Here's how the part is built. I have some questions about the finished solid (model axes, mm). A direction names the side the tool comes from. Coordinates: 2 decimals unless noted, no trailing zeros. Write each loop counter-clockwise with the first axis right and the second up, starting at its lowest first coordinate (ties: lowest second). Pieces come first, ordered by that corner, then holes.
(1) Imagine slicing it at A-A, the plane y = -10.5. List the corners of the cut face in (x, z) for me, plus the area to 3 significant figures.
(2) Thinking about a two-plate mould opening in Z: for faces 1 (the flat face through (-2, -15, 5)), 2 (the flat face through (-2, -7, 373)), 3 (the flat face through (117, -5, 114)), which applies, released by +Z, released by -Z, zero draft, split by the parting line, or undercut?
(3) Which directions (+Z, -Z, +X, -X, +Y, -Y) give clear straight access to the entire face, cutting with the end or side of a thin tool? Please do faces 4 (the flat face through (-2, 0, 5)), 5 (the cylindrical face through (117.7, -10.1, 48)).
(4) Please list where these lines run through material, in increasing order: probe 1 along Z at (x, y) = (126, -11.25); probe 2 along X at (y, z) = (-10.5, 58).
(5) For pin 1 Ø8 at (x, z) = (-51.5, 65.5) entering from +Y, with a flat end and sliding along its axis, tell me the tip position at first contact or that it passes through.
(6) Imagine slicing it at B-B, the plane x = 117.5. List the corners of the cut face in (y, z) for me, plus the area to 3 significant figures.
```python
from build123d import *

# Parameters (mm, degrees)
F0_W     = 295
F0_H     = 746
F1_DEPTH = 15
F3_DEPTH = 10


with BuildPart() as f1:
    # F0 (on Front) → F1 (new body)
    with BuildSketch(Plane.XZ):
        Rectangle(F0_W, F0_H)
    extrude(amount=F1_DEPTH)

    # F2 (on face) → F3 (cut)
    with BuildSketch(Plane.XZ.offset(15)):
        with BuildLine():
            ThreePointArc((132.4401133717, 161.6609658553), (132.4850208638, 162.3298136735), (132.5, 163))
            ThreePointArc((132.5, 163), (116.3496874374, 177.9558276604), (102.6764291989, 160.7061498078))
            ThreePointArc((102.6764291989, 160.7061498078), (117.9809511033, 148.0077124482), (132.4401133717, 161.6609658553))
        make_face()
        with BuildLine():
            ThreePointArc((132.4401133717, 161.6609658553), (117.9809511033, 148.0077124482), (102.6764291989, 160.7061498078))
            Line((102.6764291989, 160.7061498078), (102.6764291989, 65.2938501922))
            ThreePointArc((102.6764291989, 65.2938501922), (117.9809511033, 77.9922875518), (132.4401133717, 64.3390341447))
            Line((132.4401133717, 64.3390341447), (132.4401133717, 161.6609658553))
        make_face()
        with BuildLine():
            ThreePointArc((132.4401133717, 64.3390341447), (117.9809511033, 77.9922875518), (102.6764291989, 65.2938501922))
            Line((102.6764291989, 65.2938501922), (102.6764291989, 60.7061498078))
            ThreePointArc((102.6764291989, 60.7061498078), (117.9809511033, 48.0077124482), (132.4401133717, 61.6609658553))
            Line((132.4401133717, 61.6609658553), (132.4401133717, 64.3390341447))
        make_face()
    extrude(amount=-F3_DEPTH, mode=Mode.SUBTRACT)


solid = f1.part
```
Recorded:
1. outline: (-147.5, -373) - (147.5, -373) - (147.5, 373) - (-147.5, 373) - close; hole (102.68, 60.71) arc R15 ccw to (132.44, 61.66) - (132.44, 161.66) arc R15 ccw (long way) to (102.68, 160.71) - close
1. area: 216,000 mm2
2. face 1: zero draft
2. face 2: released by +Z
2. face 3: undercut
3. face 4: +Z, -Z, +X, -X, +Y
3. face 5: -Y
4. probe 1: z = -373 to 50.64, 175.36 to 373
4. probe 2: x = -147.5 to 103.36, 131.64 to 147.5
5. pin 1: stops at y = 0
6. outline: (-15, -373) - (0, -373) - (0, 373) - (-15, 373) - (-15, 178) - (-5, 178) - (-5, 48) - (-15, 48) - close
6. area: 9,890 mm2
